Verification items for the finished model (mm, model axes). A direction names the side the tool comes from. Round coordinates to 2 decimals unless told otherwise and drop trailing zeros. Order: outer loops, then holes, each group sorted by start corner. A loop starts at its lowest first (then second) coordinate and runs counter-clockwise, first axis right, second up. Notation, with made-up numbers: (25.5, 71.5) -> (59.5, 71.5) arc R20 cw to (59.5, 109.5) -> close; hole circle Ø8 at (-38.75, 8). An arc over 180 degrees is marked (long way). Put each result on its own line as item: value.
```python
from build123d import *

# Parameters (mm, degrees)
F1_DEPTH = 31.75
F2_R     = 5.08
F4_D     = 8.73252


with BuildPart() as f1:
    # F0 (on Front) → F1 (new body)
    with BuildSketch(Plane.XZ):
        Polygon((0, -6.35), (0, 0), (-5.08, 0), (-5.08, 9.652), (-41.275, 9.652), (-41.275, 0), (-41.275, -6.35), align=None)
    extrude(amount=F1_DEPTH)

    # F2
    f2_edges = [f1.edges().sort_by_distance(p)[0] for p in [
        (-41.275, -31.75, 1.651),
        (-41.275, 0, 1.651),
    ]]
    fillet(f2_edges, radius=F2_R)

    # F4 (through all)
    with Locations(Plane(origin=(0, 0, -6.35), x_dir=(1, 0, 0), z_dir=(0, 0, -1))):
        with Locations((-31.75, 15.875)):
            Hole(F4_D / 2)

    # F5: F1 across plane


with BuildPart() as f1_1:
    add(f1.part)
    add(f1.part.mirror(Plane.YZ))


solid = f1_1.part
```
Item 1: Sectioned sample at B-B, the plane x = 31.75. Record the boundary of the cut face in (y, z), then the cut area to 3 significant figures.
Geometry check:
outline: (-31.75, -6.35) -> (-20.24, -6.35) -> (-20.24, 9.65) -> (-31.75, 9.65) -> close; (-11.51, -6.35) -> (0, -6.35) -> (0, 9.65) -> (-11.51, 9.65) -> close
area: 368 mm2
Item 2: Sectioned sample at A-A, the plane z = 1.75. Record the boundary of the cut face in (x, y) (3 decimals), then the cut area to 3 significant figures.
Geometry check:
outline: (-41.275, -26.67) arc R5.08 ccw to (-36.195, -31.75) -> (-5.08, -31.75) -> (-5.08, 0) -> (-36.195, 0) arc R5.08 ccw to (-41.275, -5.08) -> close; (5.08, -31.75) -> (36.195, -31.75) arc R5.08 ccw to (41.275, -26.67) -> (41.275, -5.08) arc R5.08 ccw to (36.195, 0) -> (5.08, 0) -> close; hole circle Ø8.733 at (-31.75, -15.875); hole circle Ø8.733 at (31.75, -15.875)
area: 2,160 mm2
Item 3: Depth check by flat-ended pin: pin 1 Ø8 at (x, y) = (31.75, -15.875) entering from -Z; pin 2 Ø8 at (x, y) = (0.5, -22.5) entering from +Z. Enter the tip coordinate at first touch or a pass-through.
Geometry check:
pin 1: through
pin 2: z = 0
Item 4: Release check for a two-part mould opening along Y. For faces 1 (the face through (39.8, -1.5, 1.5)), 2 (the face through (-41.275, -16, 2)), 3 (the face through (28.532, -18.826, 1.763)) record: pulls with the +Y half, pulls with the -Y half, needs draft (parallel to the pull), parting line crosses it, or undercut.
Geometry check:
face 1: pulls with the +Y half
face 2: needs draft
face 3: undercut
Item 5: Sectioned sample at D-D, the plane y = -18. Record the boundary of the cut face in (x, z) (3 decimals).
Geometry check:
outline: (-41.275, -6.35) -> (-35.564, -6.35) -> (-35.564, 9.652) -> (-41.275, 9.652) -> close; (-27.936, -6.35) -> (27.936, -6.35) -> (27.936, 9.652) -> (5.08, 9.652) -> (5.08, 0) -> (-5.08, 0) -> (-5.08, 9.652) -> (-27.936, 9.652) -> close; (35.564, -6.35) -> (41.275, -6.35) -> (41.275, 9.652) -> (35.564, 9.652) -> close
Item 6: Material ranges on line 1 along Y through (x, z) = (-31.75, 4.5); line 2 along X through (y, z) = (-12, -2) (3 decimals); line 3 along X through (y, z) = (-22.5, 4.25) (3 decimals), recorded low to high.
Geometry check:
line 1: -31.75 to -20.24, -11.51 to 0
line 2: -41.275 to -33.762, -29.738 to 29.738, 33.762 to 41.275
line 3: -41.275 to -5.08, 5.08 to 41.275
Item 7: Tool access check on faces 4 (the face through (39.83, -30.22, 1.54)), 5 (the face through (-5.08, -16, 5)). Record the directions out of +Z, -Z, +X, -X, +Y, -Y that give a thin tool (end or side, any length) a straight path to the whole face; none if there is none.
Geometry check:
face 4: +Z, -Z, +X, -Y
face 5: +Z, +Y, -Y
Item 8: Sectioned sample at C-C, the plane y = -7. Record the boundary of the cut face in (x, z) (3 decimals).
Geometry check:
outline: (-41.275, -6.35) -> (41.275, -6.35) -> (41.275, 9.652) -> (5.08, 9.652) -> (5.08, 0) -> (-5.08, 0) -> (-5.08, 9.652) -> (-41.275, 9.652) -> close
